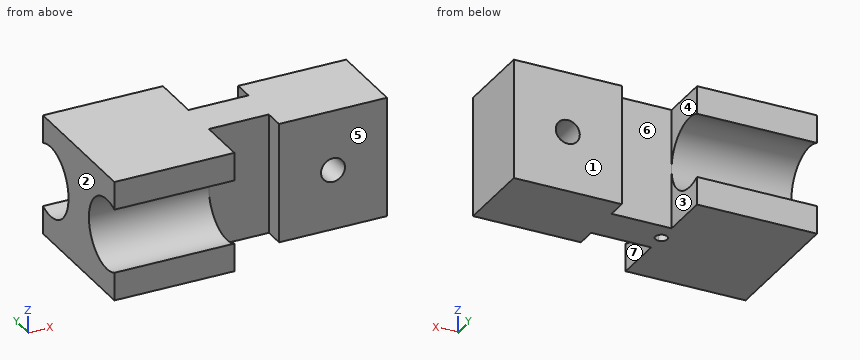
```python
from build123d import *

# Parameters (mm, degrees)
SKETCH1_W           = 30
SKETCH1_H           = 35
SKETCH1_W_2         = 27
SKETCH1_H_2         = 20
SKETCH1_W_3         = 15
SKETCH1_H_3         = 10
BOSS_EXTRUDE1_DEPTH = 30
CUT_EXTRUDE1_DEPTH  = 8
SKETCH15_R          = 3
CUT_EXTRUDE3_DEPTH  = 71.037489961
CUT_EXTRUDE6_DEPTH  = 30


with BuildPart() as part:
    # Sketch1 → Boss-Extrude1 (new body)
    with BuildSketch(Plane.XY):
        Rectangle(SKETCH1_W, SKETCH1_H)
        with Locations((43.5, 0)):
            Rectangle(SKETCH1_W_2, SKETCH1_H_2)
        with Locations((22.5, 0)):
            Rectangle(SKETCH1_W_3, SKETCH1_H_3)
    extrude(amount=BOSS_EXTRUDE1_DEPTH)

    # Sketch1<3> → Cut-Extrude1 (cut)
    with BuildSketch(Plane.XY):
        with BuildLine():
            ThreePointArc((15, 1.5), (13.5, 0), (15, -1.5))
            Line((15, -1.5), (15, 1.5))
        make_face()
        with BuildLine():
            Line((15, 1.5), (15, -1.5))
            ThreePointArc((15, -1.5), (16.060660172, -1.060660172), (16.5, 0))
            ThreePointArc((16.5, 0), (16.060660172, 1.060660172), (15, 1.5))
        make_face()
    extrude(amount=CUT_EXTRUDE1_DEPTH, mode=Mode.SUBTRACT)

    # Sketch15 → Cut-Extrude3 (cut, through all)
    with BuildSketch(Plane(origin=(0, 10, 0), x_dir=(1, 0, 0), z_dir=(0, 1, 0))):
        with Locations(Location((43.5, -15, 0), (0, 0, 270))):
            Circle(SKETCH15_R)
    extrude(amount=-CUT_EXTRUDE3_DEPTH, mode=Mode.SUBTRACT)

    # Sketch5 → Cut-Extrude6 (cut)
    with BuildSketch(Plane.ZY.offset(15)):
        with BuildLine():
            Line((7, -17.5), (23, -17.5))
            ThreePointArc((23, -17.5), (15, -5), (7, -17.5))
        make_face()
        with BuildLine():
            Line((7, 17.5), (23, 17.5))
            ThreePointArc((23, 17.5), (15, 5), (7, 17.5))
        make_face()
    extrude(amount=-CUT_EXTRUDE6_DEPTH, mode=Mode.SUBTRACT)


solid = part.part
```
CAD build for the part. Positions are in the model's coordinates, mm. Face numbers are marked on the shaded views. A direction names the side the tool comes from. Coordinates: 2 decimals unless noted, no trailing zeros. Write each loop counter-clockwise with the first axis right and the second up, starting at its lowest first coordinate (ties: lowest second). Pieces come first, ordered by that corner, then holes. Notation, with made-up numbers: (26.5, 43) -> (57.5, 43) arc R31 ccw to (57.5, 75) -> close; hole circle Ø11 at (-33.5, 89.25). An arc over 180 degrees is marked (long way). Return JSON: item names as keys, results as strings. Group by question number.
Q1. Cut at D-D, the plane z = 12.75. Give the cut face in (x, y).
Q2. Cut at A-A, the plane x = 43.5. Give the cut face in (y, z), then the cut area to 3 significant figures.
Q3. Pull direction X, two halves, no side cores. Call the marked faces 1, 2, 3 and 4: released by +X, released by -X, zero draft, split by the parting line, or undercut.
Q4. Which spindle directions (+Z, -Z, +X, -X, +Y, -Y) get a long thin tool onto all of the face, cutting with end or side? Do the marked faces 5, 6 and 7. Say none if no direction does.
Q5. Cut at C-C, the plane x = -0.5. Give the cut face in (y, z).
Q6. Flat gauge pins, fed straight in: pin 1 (2.5 mm diameter, centred on x = 15, y = 0.5, fed in from -Z); pin 2 (1 mm diameter, centred on x = 19, z = 25, fed in from +Y); pin 3 (2.5 mm diameter, centred on y = 8, z = 12.5, fed in from -X); pin 4 (12 mm diameter, centred on x = 25.5, z = 18.5, fed in from +Y). Where does each tip first touch, or does it go through?
Q7. Cut at B-B, the plane y = -13.81. Give the cut face in (x, z).
Q8. Drill centre lines: line 1 (Z direction, x = -7, y = -13.81); line 2 (X direction, y = 7.5, z = 25); line 3 (X direction, y = 6.25, z = 15). Where is each one in solid material? Low to high.
Returned:
{
 "1": {"outline": "(-15, -5.29) -> (15, -5.29) -> (15, -5) -> (30, -5) -> (30, -10) -> (41.52, -10) -> (41.52, 10) -> (30, 10) -> (30, 5) -> (15, 5) -> (15, 5.29) -> (-15, 5.29) -> close; (45.48, -10) -> (57, -10) -> (57, 10) -> (45.48, 10) -> close"},
 "2": {"outline": "(-10, 0) -> (10, 0) -> (10, 12) -> (-10, 12) -> close; (-10, 18) -> (10, 18) -> (10, 30) -> (-10, 30) -> close", "area": "480 mm2"},
 "3": {"face 1": "zero draft", "face 2": "released by -X", "face 3": "undercut", "face 4": "undercut"},
 "4": {"face 5": "+Z, -Z, +X, -Y", "face 6": "+Z, -Z, +Y", "face 7": "+Z, -Z, -Y"},
 "5": {"outline": "(-17.5, 0) -> (17.5, 0) -> (17.5, 7) arc R8.81 cw (long way) to (17.5, 23) -> (17.5, 30) -> (-17.5, 30) -> (-17.5, 23) arc R8.81 cw (long way) to (-17.5, 7) -> close"},
 "6": {"pin 1": "stops at z = 0", "pin 2": "stops at y = 5", "pin 3": "stops at x = 30", "pin 4": "stops at y = 10"},
 "7": {"outline": "(-15, 0) -> (15, 0) -> (15, 6.19) -> (-15, 6.19) -> close; (-15, 23.81) -> (15, 23.81) -> (15, 30) -> (-15, 30) -> close"},
 "8": {"line 1": "z = 0 to 6.19, 23.81 to 30", "line 2": "x = -15 to 15, 30 to 57", "line 3": "x = 30 to 40.5, 46.5 to 57"}
}
